Could you check a few things on this drawing? It's one solid part, dimensions in mm from its lowest x, y, z. Round coordinates to 2 decimals unless told otherwise and drop trailing zeros. Order: outer loops, then holes, each group sorted by start corner. A loop starts at its lowest first (then second) coordinate and runs counter-clockwise, first axis right, second up.
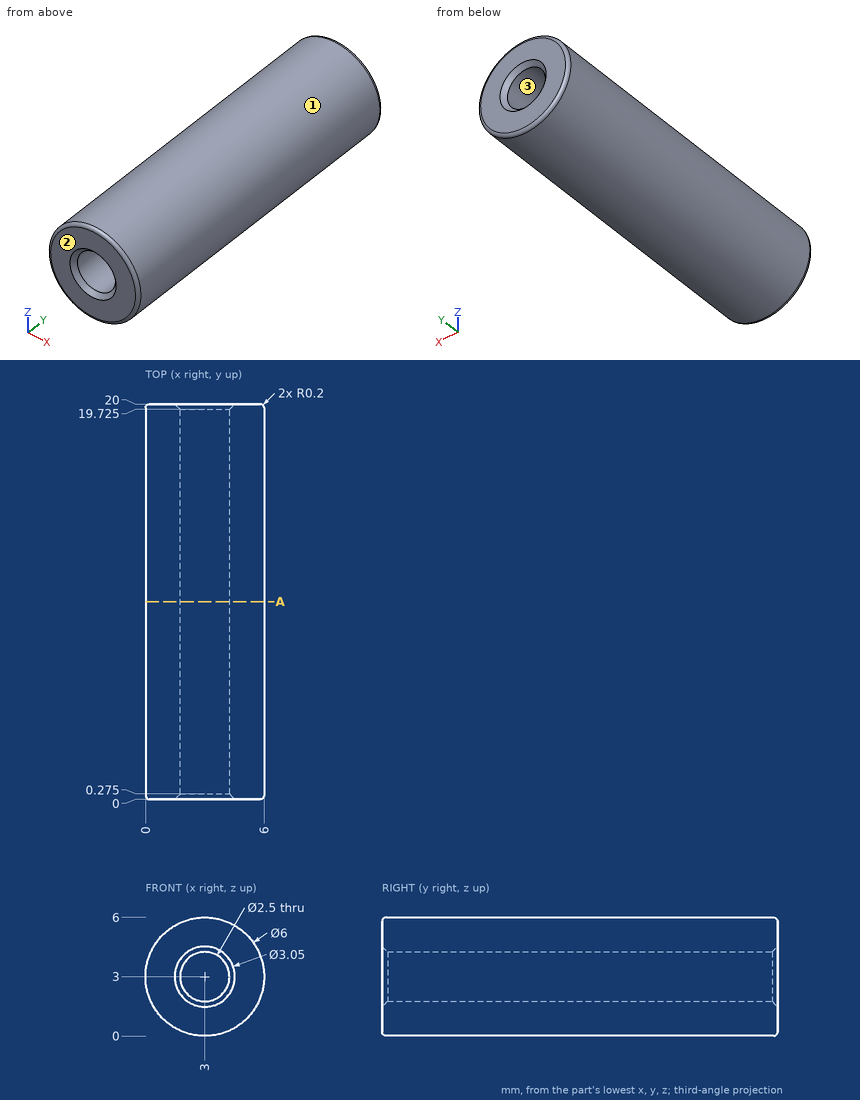
1) We'd pull the mould along X, two halves only. Please class the marked faces 1, 2 and 3: +X half, -X half, draft (parallel to the pull), parting line (faces both ways), or undercut.
2) If we section it at A-A (y = 10): Write out the boundary of the cut face in (x, z), plus the area to 3 significant figures.
3) I need wall thicknesses on line 1 (X direction, y = 4.75, z = 3); line 2 (Z direction, x = 3.5, y = 14). Which ranges of each line are inside material? Lowest first, please.
Solutions:
1. face 1: parting line
1. face 2: draft
1. face 3: undercut
2. outline: circle Ø6 at (3, 3); hole circle Ø2.5 at (3, 3)
2. area: 23.4 mm2
3. line 1: x = 0 to 1.75, 4.25 to 6
3. line 2: z = 0.04 to 1.85, 4.15 to 5.96
